```python
from build123d import *

# Parameters (mm, degrees)
SKETCH1_W           = 200
SKETCH1_H           = 50
BOSS_EXTRUDE1_DEPTH = 3
SKETCH2_W           = 20
SKETCH2_H           = 3
SKETCH2_W_2         = 3
SKETCH2_H_2         = 10
CUT_EXTRUDE1_DEPTH  = 3
CUT_EXTRUDE2_DEPTH  = 3


with BuildPart() as part:
    # Sketch1 → Boss-Extrude1 (new body)
    with BuildSketch(Plane.XY):
        Rectangle(SKETCH1_W, SKETCH1_H)
    extrude(amount=BOSS_EXTRUDE1_DEPTH)

    # Sketch2 → Cut-Extrude1 (cut)
    with BuildSketch(Plane.XY.offset(3)):
        with Locations((-70, 23.5)):
            Rectangle(SKETCH2_W, SKETCH2_H)
        with Locations((-30, -23.5)):
            Rectangle(SKETCH2_W, SKETCH2_H)
        with Locations((98.5, 0)):
            Rectangle(SKETCH2_W_2, SKETCH2_H_2)
        with Locations((-70, -23.5)):
            Rectangle(SKETCH2_W, SKETCH2_H)
        with Locations((30, 23.5)):
            Rectangle(SKETCH2_W, SKETCH2_H)
        with Locations((70, 23.5)):
            Rectangle(SKETCH2_W, SKETCH2_H)
        with Locations((-30, 23.5)):
            Rectangle(SKETCH2_W, SKETCH2_H)
        with Locations((30, -23.5)):
            Rectangle(SKETCH2_W, SKETCH2_H)
        with Locations((70, -23.5)):
            Rectangle(SKETCH2_W, SKETCH2_H)
        with Locations((-98.5, 0)):
            Rectangle(SKETCH2_W_2, SKETCH2_H_2)
    extrude(amount=-CUT_EXTRUDE1_DEPTH, mode=Mode.SUBTRACT)

    # Sketch3 → Cut-Extrude2 (cut)
    with BuildSketch(Plane.XY.offset(3)):
        with BuildLine():
            Line((75, 7.5), (-75, 7.5))
            ThreePointArc((-75, 7.5), (-77.5, 10), (-75, 12.5))
            Line((-75, 12.5), (75, 12.5))
            ThreePointArc((75, 12.5), (77.5, 10), (75, 7.5))
        make_face()
        with BuildLine():
            Line((75, -2.5), (-75, -2.5))
            ThreePointArc((-75, -2.5), (-77.5, 0), (-75, 2.5))
            Line((-75, 2.5), (75, 2.5))
            ThreePointArc((75, 2.5), (77.5, 0), (75, -2.5))
        make_face()
        with BuildLine():
            Line((75, -12.5), (-75, -12.5))
            ThreePointArc((-75, -12.5), (-77.5, -10), (-75, -7.5))
            Line((-75, -7.5), (75, -7.5))
            ThreePointArc((75, -7.5), (77.5, -10), (75, -12.5))
        make_face()
    extrude(amount=-CUT_EXTRUDE2_DEPTH, mode=Mode.SUBTRACT)


solid = part.part
```
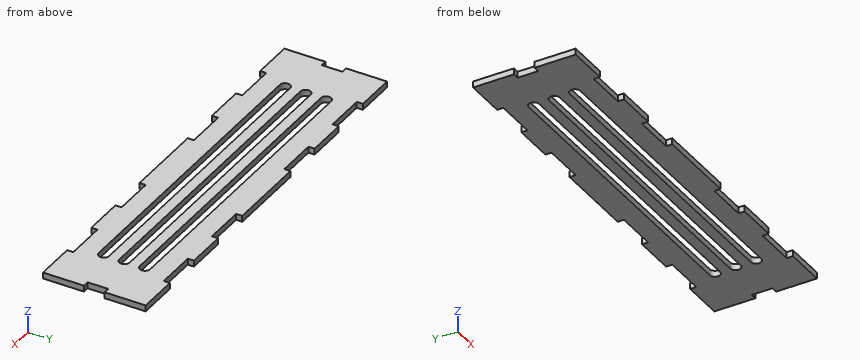
Could you check a few things on this model? Use its own coordinates, in mm. Coordinates: 2 decimals unless noted, no trailing zeros. Write each loop counter-clockwise with the first axis right and the second up, starting at its lowest first coordinate (ties: lowest second). Pieces come first, ordered by that corner, then holes. Notation, with made-up numbers: (20, 5) -> (37, 5) arc R26 ccw to (37, 22) -> close; hole circle Ø10 at (2, 47). An arc over 180 degrees is marked (long way). Return JSON: item names as keys, results as strings.
(1) I need wall thicknesses on L1, parallel to Y at x = 45.5, z = 2.3; L2, parallel to Y at x = -62.5, z = 1.95; L3, parallel to X at y = 3, z = 2. Which ranges of each line are inside material? Lowest first, please.
Numbers:
{"L1": "y = -25 to -12.5, -7.5 to -2.5, 2.5 to 7.5, 12.5 to 25", "L2": "y = -22 to -12.5, -7.5 to -2.5, 2.5 to 7.5, 12.5 to 22", "L3": "x = -97 to 97"}
(2) Imagine slicing it at D-D, the plane y = 10. Please give me the cut outline in (x, z), then the cut area to 3 significant figures.
Numbers:
{"outline": "(-100, 0) -> (-77.5, 0) -> (-77.5, 3) -> (-100, 3) -> close; (77.5, 0) -> (100, 0) -> (100, 3) -> (77.5, 3) -> close", "area": "135 mm2"}
(3) I'm going to push a flat-ended pin straight in: pin 1 (1.5 mm diameter, centred on x = 37, z = 1, fed in from -Y). Where does the tip first touch, or does it pass through?
Numbers:
{"pin 1": "stops at y = -22"}
(4) Imagine slicing it at A-A, the plane x = -45.5. Please give me the cut outline in (y, z).
Numbers:
{"outline": "(-25, 0) -> (-12.5, 0) -> (-12.5, 3) -> (-25, 3) -> close; (-7.5, 0) -> (-2.5, 0) -> (-2.5, 3) -> (-7.5, 3) -> close; (2.5, 0) -> (7.5, 0) -> (7.5, 3) -> (2.5, 3) -> close; (12.5, 0) -> (25, 0) -> (25, 3) -> (12.5, 3) -> close"}
(5) Imagine slicing it at C-C, the plane z = 1. Count the separate pieces of the cut face and the enclosed holes in it, then the cut area to 3 significant figures.
Numbers:
{"separate pieces": "1", "enclosed holes": "3", "area": "7,150 mm2"}
(6) Imagine slicing it at B-B, the plane y = 0. Please give me the cut outline in (x, z).
Numbers:
{"outline": "(-97, 0) -> (-77.5, 0) -> (-77.5, 3) -> (-97, 3) -> close; (77.5, 0) -> (97, 0) -> (97, 3) -> (77.5, 3) -> close"}
